from build123d import *

# Parameters (mm, degrees)
F0_W     = 10
F0_H     = 10
F0_R     = 0.55
F0_R_2   = 1.537619
F1_DEPTH = 2
F2_DEPTH = 1


with BuildPart() as f1:
    # F0 (on Top) → F1 (new body)
    with BuildSketch(Plane.XY):
        Rectangle(F0_W, F0_H)
        with Locations((-4, -4)):
            Circle(F0_R, mode=Mode.SUBTRACT)
        with Locations((4, -4)):
            Circle(F0_R, mode=Mode.SUBTRACT)
        with Locations((-4, 4)):
            Circle(F0_R, mode=Mode.SUBTRACT)
        with BuildLine():
            ThreePointArc((-3.213514, -2.50617), (-2.881628, 2.881628), (2.50617, 3.213514))
            Line((2.50617, 3.213514), (3.235023, 3.942367))
            Line((3.235023, 3.942367), (3.603887, 3.573503))
            Line((3.603887, 3.573503), (3.942129, 3.23526))
            Line((3.942129, 3.23526), (3.213306, 2.506437))
            ThreePointArc((3.213306, 2.506437), (2.881628, -2.881628), (-2.506437, -3.213306))
            Line((-2.506437, -3.213306), (-3.23526, -3.942129))
            Line((-3.23526, -3.942129), (-3.573503, -3.603887))
            Line((-3.573503, -3.603887), (-3.942367, -3.235023))
            Line((-3.942367, -3.235023), (-3.213514, -2.50617))
        make_face(mode=Mode.SUBTRACT)
        with Locations((4, 4)):
            Circle(F0_R, mode=Mode.SUBTRACT)
        with BuildLine():
            Line((3.235023, 3.942367), (2.50617, 3.213514))
            ThreePointArc((2.50617, 3.213514), (-2.881628, 2.881628), (-3.213514, -2.50617))
            Line((-3.213514, -2.50617), (-3.942367, -3.235023))
            Line((-3.942367, -3.235023), (-3.573503, -3.603887))
            Line((-3.573503, -3.603887), (-3.23526, -3.942129))
            Line((-3.23526, -3.942129), (-2.506437, -3.213306))
            ThreePointArc((-2.506437, -3.213306), (2.881628, -2.881628), (3.213306, 2.506437))
            Line((3.213306, 2.506437), (3.942129, 3.23526))
            Line((3.942129, 3.23526), (3.603887, 3.573503))
            Line((3.603887, 3.573503), (3.235023, 3.942367))
        make_face()
        with BuildLine():
            Line((-3.034318, -0.5), (-2.526232, -0.5))
            ThreePointArc((-2.526232, -0.5), (-1.820968, -1.820968), (-0.5, -2.526232))
            Line((-0.5, -2.526232), (-0.5, -3.034318))
            ThreePointArc((-0.5, -3.034318), (-2.174521, -2.174521), (-3.034318, -0.5))
        make_face(mode=Mode.SUBTRACT)
        with BuildLine():
            ThreePointArc((0.5, -2.526232), (1.820968, -1.820968), (2.526232, -0.5))
            Line((2.526232, -0.5), (3.034318, -0.5))
            ThreePointArc((3.034318, -0.5), (2.174521, -2.174521), (0.5, -3.034318))
            Line((0.5, -3.034318), (0.5, -2.526232))
        make_face(mode=Mode.SUBTRACT)
        with BuildLine():
            ThreePointArc((-0.5, 2.526232), (-1.820968, 1.820968), (-2.526232, 0.5))
            Line((-2.526232, 0.5), (-3.034318, 0.5))
            ThreePointArc((-3.034318, 0.5), (-2.174521, 2.174521), (-0.5, 3.034318))
            Line((-0.5, 3.034318), (-0.5, 2.526232))
        make_face(mode=Mode.SUBTRACT)
        Circle(F0_R_2, mode=Mode.SUBTRACT)
        with BuildLine():
            Line((3.034318, 0.5), (2.526232, 0.5))
            ThreePointArc((2.526232, 0.5), (1.820968, 1.820968), (0.5, 2.526232))
            Line((0.5, 2.526232), (0.5, 3.034318))
            ThreePointArc((0.5, 3.034318), (2.174521, 2.174521), (3.034318, 0.5))
        make_face(mode=Mode.SUBTRACT)
        with BuildLine():
            ThreePointArc((-0.5, -2.526232), (-1.820968, -1.820968), (-2.526232, -0.5))
            Line((-2.526232, -0.5), (-3.034318, -0.5))
            ThreePointArc((-3.034318, -0.5), (-2.174521, -2.174521), (-0.5, -3.034318))
            Line((-0.5, -3.034318), (-0.5, -2.526232))
        make_face()
        with BuildLine():
            Line((-3.034318, 0.5), (-2.526232, 0.5))
            ThreePointArc((-2.526232, 0.5), (-1.820968, 1.820968), (-0.5, 2.526232))
            Line((-0.5, 2.526232), (-0.5, 3.034318))
            ThreePointArc((-0.5, 3.034318), (-2.174521, 2.174521), (-3.034318, 0.5))
        make_face()
        with BuildLine():
            ThreePointArc((0.5, 2.526232), (1.820968, 1.820968), (2.526232, 0.5))
            Line((2.526232, 0.5), (3.034318, 0.5))
            ThreePointArc((3.034318, 0.5), (2.174521, 2.174521), (0.5, 3.034318))
            Line((0.5, 3.034318), (0.5, 2.526232))
        make_face()
        with BuildLine():
            Line((3.034318, -0.5), (2.526232, -0.5))
            ThreePointArc((2.526232, -0.5), (1.820968, -1.820968), (0.5, -2.526232))
            Line((0.5, -2.526232), (0.5, -3.034318))
            ThreePointArc((0.5, -3.034318), (2.174521, -2.174521), (3.034318, -0.5))
        make_face()
        Circle(F0_R_2)
    extrude(amount=-F1_DEPTH)

    # F0 (on Top) → F2 (cut)
    with BuildSketch(Plane.XY):
        with BuildLine():
            Line((3.235023, 3.942367), (2.50617, 3.213514))
            ThreePointArc((2.50617, 3.213514), (-2.881628, 2.881628), (-3.213514, -2.50617))
            Line((-3.213514, -2.50617), (-3.942367, -3.235023))
            Line((-3.942367, -3.235023), (-3.573503, -3.603887))
            Line((-3.573503, -3.603887), (-3.23526, -3.942129))
            Line((-3.23526, -3.942129), (-2.506437, -3.213306))
            ThreePointArc((-2.506437, -3.213306), (2.881628, -2.881628), (3.213306, 2.506437))
            Line((3.213306, 2.506437), (3.942129, 3.23526))
            Line((3.942129, 3.23526), (3.603887, 3.573503))
            Line((3.603887, 3.573503), (3.235023, 3.942367))
        make_face()
        with BuildLine():
            Line((-3.034318, -0.5), (-2.526232, -0.5))
            ThreePointArc((-2.526232, -0.5), (-1.820968, -1.820968), (-0.5, -2.526232))
            Line((-0.5, -2.526232), (-0.5, -3.034318))
            ThreePointArc((-0.5, -3.034318), (-2.174521, -2.174521), (-3.034318, -0.5))
        make_face(mode=Mode.SUBTRACT)
        with BuildLine():
            ThreePointArc((0.5, -2.526232), (1.820968, -1.820968), (2.526232, -0.5))
            Line((2.526232, -0.5), (3.034318, -0.5))
            ThreePointArc((3.034318, -0.5), (2.174521, -2.174521), (0.5, -3.034318))
            Line((0.5, -3.034318), (0.5, -2.526232))
        make_face(mode=Mode.SUBTRACT)
        with BuildLine():
            ThreePointArc((-0.5, 2.526232), (-1.820968, 1.820968), (-2.526232, 0.5))
            Line((-2.526232, 0.5), (-3.034318, 0.5))
            ThreePointArc((-3.034318, 0.5), (-2.174521, 2.174521), (-0.5, 3.034318))
            Line((-0.5, 3.034318), (-0.5, 2.526232))
        make_face(mode=Mode.SUBTRACT)
        Circle(F0_R_2, mode=Mode.SUBTRACT)
        with BuildLine():
            Line((3.034318, 0.5), (2.526232, 0.5))
            ThreePointArc((2.526232, 0.5), (1.820968, 1.820968), (0.5, 2.526232))
            Line((0.5, 2.526232), (0.5, 3.034318))
            ThreePointArc((0.5, 3.034318), (2.174521, 2.174521), (3.034318, 0.5))
        make_face(mode=Mode.SUBTRACT)
    extrude(amount=-F2_DEPTH, mode=Mode.SUBTRACT)


solid = f1.part
Work out the finished part from the listing and answer in its coordinate system (mm). A direction names the side the tool comes from. Coordinates: 2 decimals unless noted, no trailing zeros. Write each loop counter-clockwise with the first axis right and the second up, starting at its lowest first coordinate (ties: lowest second). Pieces come first, ordered by that corner, then holes.
1. A flat-ended cylindrical pin translates along its axis: pin 1 (6 mm diameter, centred on x = -1.5, y = -2.5, fed in from +Z). Find the tip coordinate at first contact, or state that the pin passes through.
Results list:
pin 1: stops at z = 0
2. For faces 3 (the cylindrical face through (-3.49, 3.79, -0.99)), 4 (the cylindrical face through (1.806, -1.836, -0.493)), determine the directions among +Z, -Z, +X, -X, +Y, -Y from which every point of the face is accessible in a straight line to the end or side of a thin tool.
Results list:
face 3: +Z, -Z
face 4: +Z
3. The part is cut by section A-A, the plane z = -1.45. Write down the section's boundary in (x, y), and give its area (3 significant figures).
Results list:
outline: (-5, -5) - (5, -5) - (5, 5) - (-5, 5) - close; hole circle Ø1.1 at (-4, -4); hole circle Ø1.1 at (-4, 4); hole circle Ø1.1 at (4, -4); hole circle Ø1.1 at (4, 4)
area: 96.2 mm2
4. The part is cut by section D-D, the plane y = 2.25. Write down the section's boundary in (x, z).
Results list:
outline: (-5, -2) - (5, -2) - (5, 0) - (3.4, 0) - (3.4, -1) - (2.1, -1) - (2.1, 0) - (1.25, 0) - (1.25, -1) - (-1.25, -1) - (-1.25, 0) - (-2.1, 0) - (-2.1, -1) - (-3.4, -1) - (-3.4, 0) - (-5, 0) - close
5. Consider line 1 along Y through (x, z) = (-4, -1.2); line 2 along Y through (x, z) = (1.25, -0.45); line 3 along Y through (x, z) = (2, -0.5). Determine where each line is inside the solid, lowest interval first.
Results list:
line 1: y = -5 to -4.55, -3.45 to 3.45, 4.55 to 5
line 2: y = -5 to -3.88, -2.81 to -2.25, -0.9 to 0.9, 2.25 to 2.81, 3.88 to 5
line 3: y = -5 to -3.55, -2.34 to -1.62, 1.62 to 2.34, 3.55 to 5
6. The part is cut by section B-B, the plane x = 0. Write down the section's boundary in (y, z).
Results list:
outline: (-5, -2) - (5, -2) - (5, 0) - (4.08, 0) - (4.08, -1) - (1.54, -1) - (1.54, 0) - (-1.54, 0) - (-1.54, -1) - (-4.08, -1) - (-4.08, 0) - (-5, 0) - close
7. For a pull along X with two mould halves and no side action, classify faces 1 (the flat face through (0, -5, -1)), 2 (the cylindrical face through (2.16, 2.19, -0.49)) as +X half, -X half, draft (parallel to the pull), parting line (faces both ways), or undercut.
Results list:
face 1: draft
face 2: undercut
